Build history of the part. All positions in model axes, mm. Face numbers are marked on the shaded views. A direction names the side the tool comes from. Round coordinates to 2 decimals unless told otherwise and drop trailing zeros. Write each loop counter-clockwise with the first axis right and the second up, starting at its lowest first coordinate (ties: lowest second). Pieces come first, ordered by that corner, then holes. Notation, with made-up numbers: M 11.5,88.25 L 65.5,88.25 A18 ccw 65.5,96.25 Z; hole C -16,55.25 d8. An arc over 180 degrees is marked long. Use a Markdown table: item, result.
from build123d import *

# Parameters (mm, degrees)
SKETCH1_W           = 7
SKETCH1_H           = 7
BOSS_EXTRUDE1_DEPTH = 3
CUT_EXTRUDE1_DEPTH  = 7
CUT_EXTRUDE2_DEPTH  = 11
SKETCH4_R           = 1.8
CUT_EXTRUDE3_DEPTH  = 0.8
CUT_EXTRUDE4_DEPTH  = 0.4


with BuildPart() as part:
    # Sketch1 → Boss-Extrude1 (new body)
    with BuildSketch(Plane(origin=(0, 0, 0), x_dir=(1, 0, 0), z_dir=(0, 1, 0))):
        with Locations((3.5, 3.5)):
            Rectangle(SKETCH1_W, SKETCH1_H)
    extrude(amount=BOSS_EXTRUDE1_DEPTH)

    # Sketch2 → Cut-Extrude1 (cut)
    with BuildSketch(Plane.XY):
        Polygon((0, 0), (0.7, 3), (0, 3), align=None)
        Polygon((7, 0), (6.3, 3), (7, 3), align=None)
    extrude(amount=-CUT_EXTRUDE1_DEPTH, mode=Mode.SUBTRACT)

    # Sketch3 → Cut-Extrude2 (cut)
    with BuildSketch(Plane(origin=(0, 0, 0), x_dir=(0, 0, -1), z_dir=(1, 0, 0))):
        Polygon((0, 0), (0.7, 3), (0, 3), align=None)
        Polygon((7, 3), (6.3, 3), (7, 0), align=None)
    extrude(amount=CUT_EXTRUDE2_DEPTH, mode=Mode.SUBTRACT)

    # Sketch4 → Cut-Extrude3 (cut)
    with BuildSketch(Plane.XZ):
        with Locations(Location((3.5, -3.5, 0), (0, 0, 270))):
            Circle(SKETCH4_R)
    extrude(amount=-CUT_EXTRUDE3_DEPTH, mode=Mode.SUBTRACT)

    # Sketch5 → Cut-Extrude4 (cut)
    with BuildSketch(Plane(origin=(0, 3, 0), x_dir=(1, 0, 0), z_dir=(0, 1, 0))):
        Polygon((1.77651834, 1.766029319), (1.77651834, 5.266029319), (2.915140135, 5.266029319), (3.504082443, 2.878709608), (4.09302475, 5.266029319), (5.231646545, 5.266029319), (5.231646545, 1.766029319), (4.558569622, 1.766029319), (4.536133725, 4.521437973), (3.879182603, 1.766029319), (3.128982282, 1.766029319), (2.47203116, 4.521437973), (2.449595263, 1.766029319), align=None)
    extrude(amount=-CUT_EXTRUDE4_DEPTH, mode=Mode.SUBTRACT)


solid = part.part
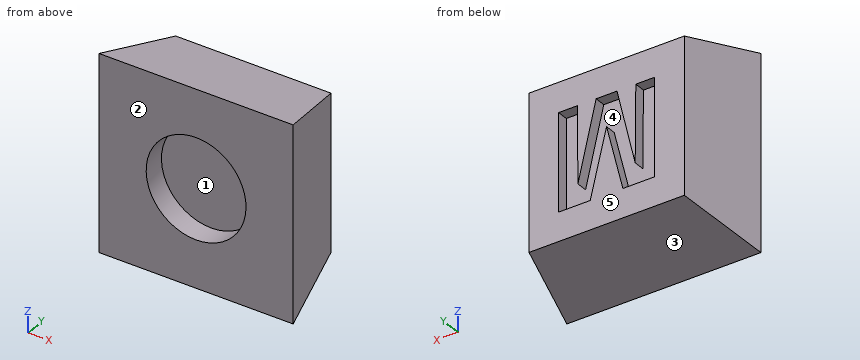
Q1. Cut at B-B on y = 2.75. Give the cut face in (x, z), and give its area (3 significant figures).
Response values:
| item | result |
|---|---|
| outline | M 0.64,-6.36 L 6.36,-6.36 L 6.36,-0.64 L 0.64,-0.64 Z; hole M 1.78,-5.27 L 2.92,-5.27 L 3.5,-2.88 L 4.09,-5.27 L 5.23,-5.27 L 5.23,-1.77 L 4.56,-1.77 L 4.54,-4.52 L 3.88,-1.77 L 3.13,-1.77 L 2.47,-4.52 L 2.45,-1.77 L 1.78,-1.77 Z |
| area | 23.9 mm2 |
Q2. Cut at D-D on z = -2.75. Give the cut face in (x, y).
Response values:
| item | result |
|---|---|
| outline | M 0,0 L 1.86,0 L 1.86,0.8 L 5.14,0.8 L 5.14,0 L 7,0 L 6.3,3 L 5.23,3 L 5.23,2.6 L 4.55,2.6 L 4.55,3 L 4.11,3 L 4.11,2.6 L 2.89,2.6 L 2.89,3 L 2.46,3 L 2.46,2.6 L 1.78,2.6 L 1.78,3 L 0.7,3 Z |
Q3. Drill centre lines: L1, parallel to Y at x = 4.25, z = -4.75; L2, parallel to X at y = 0.4, z = -2; L3, parallel to X at y = 0.5, z = -3.5. Where is each one in solid material? Low to high.
Response values:
| item | result |
|---|---|
| L1 | y = 0.8 to 2.6 |
| L2 | x = 0.09 to 2.51, 4.49 to 6.91 |
| L3 | x = 0.12 to 1.7, 5.3 to 6.88 |
Q4. Two-plate mould, pull along Z, no slides. Class the marked faces 3, 4 and 5: +Z half, -Z half, draft (parallel to the pull), parting line (faces both ways), or undercut.
Response values:
| item | result |
|---|---|
| face 3 | -Z half |
| face 4 | undercut |
| face 5 | draft |
Q5. Drop flat-ended pins along their axis: P1, Ø1, axis at y = 1.5, z = -0.5, coming from the -X side; P2, Ø1.1, axis at x = 4, z = -3, coming from the -Y side; P3, Ø1.5, axis at y = 2, z = -5.5, coming from the +X side. Give the stop position or say it passes through.
Response values:
| item | result |
|---|---|
| P1 | stops at x = 0.23 |
| P2 | stops at y = 0.8 |
| P3 | stops at x = 6.71 |
Q6. Cut at A-A on z = -5. Give the cut face in (x, y), and give its area (3 significant figures).
Response values:
| item | result |
|---|---|
| outline | M 0,0 L 2.51,0 L 2.51,0.8 L 4.49,0.8 L 4.49,0 L 7,0 L 6.3,3 L 5.23,3 L 5.23,2.6 L 4.03,2.6 L 4.03,3 L 2.98,3 L 2.98,2.6 L 1.78,2.6 L 1.78,3 L 0.7,3 Z |
| area | 16.3 mm2 |
Q7. Cut at C-C on x = 3. Give the cut face in (y, z).
Response values:
| item | result |
|---|---|
| outline | M 0,-7 L 3,-6.3 L 3,-4.92 L 2.6,-4.92 L 2.6,-2.31 L 3,-2.31 L 3,-0.7 L 0,0 L 0,-1.77 L 0.8,-1.77 L 0.8,-5.23 L 0,-5.23 Z |
Q8. Which spindle directions (+Z, -Z, +X, -X, +Y, -Y) get a long thin tool onto all of the face, cutting with end or side? Do the marked faces 1 and 2. Say none if no direction does.
Response values:
| item | result |
|---|---|
| face 1 | -Y |
| face 2 | +Z, -Z, +X, -X, -Y |
